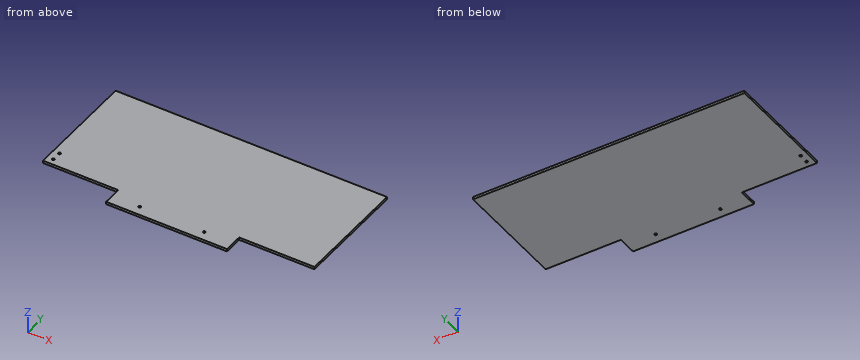
from build123d import *

# Parameters (mm, degrees)
SKETCH1_W           = 429
SKETCH1_H           = 210
BOSS_EXTRUDE1_DEPTH = 4
SKETCH2_W           = 119
SKETCH2_H           = 30
CUT_EXTRUDE1_DEPTH  = 4
SKETCH3_R           = 2
CUT_EXTRUDE2_DEPTH  = 239.854034925
SKETCH4_R           = 2
CUT_EXTRUDE3_DEPTH  = 239.854034925


with BuildPart() as part:
    # Sketch1 → Boss-Extrude1 (new body)
    with BuildSketch(Plane.XY):
        Rectangle(SKETCH1_W, SKETCH1_H)
    extrude(amount=BOSS_EXTRUDE1_DEPTH)

    # Sketch2 → Cut-Extrude1 (cut)
    with BuildSketch(Plane(origin=(0, 0, 0), x_dir=(-1, 0, 0), z_dir=(0, 0, -1))):
        with Locations((-155, -90)):
            Rectangle(SKETCH2_W, SKETCH2_H)
        with Locations((155, -90)):
            Rectangle(SKETCH2_W, SKETCH2_H)
    extrude(amount=-CUT_EXTRUDE1_DEPTH, mode=Mode.SUBTRACT)

    # Sketch3 → Cut-Extrude2 (cut, through all)
    with BuildSketch(Plane(origin=(0, 0, 0), x_dir=(-1, 0, 0), z_dir=(0, 0, -1))):
        with Locations((-49.983602513, -90)):
            Circle(SKETCH3_R)
        with Locations((52.125756906, -90)):
            Circle(SKETCH3_R)
    extrude(amount=-CUT_EXTRUDE2_DEPTH, mode=Mode.SUBTRACT)

    # Sketch4 → Cut-Extrude3 (cut, through all)
    with BuildSketch(Plane(origin=(0, 0, 0), x_dir=(-1, 0, 0), z_dir=(0, 0, -1))):
        with Locations((204.5, -65)):
            Circle(SKETCH4_R)
        with Locations((204.5, -50)):
            Circle(SKETCH4_R)
    extrude(amount=-CUT_EXTRUDE3_DEPTH, mode=Mode.SUBTRACT)


solid = part.part
Read the model definition and answer for the solid it produces. Units are mm, in the model's axes. Round coordinates to 2 decimals unless told otherwise and drop trailing zeros. Write each loop counter-clockwise with the first axis right and the second up, starting at its lowest first coordinate (ties: lowest second). Pieces come first, ordered by that corner, then holes. Notation, with made-up numbers: (87, 26.25) - (133, 26.25) arc R13 ccw to (133, 47.25) - close; hole circle Ø5 at (51.5, 52.5). An arc over 180 degrees is marked (long way). Use a Markdown table: item, result.
(1) The part is cut by section C-C (x = 151.5). Write down the section's boundary in (y, z), then the cut area to 3 significant figures.
Reported:
| item | result |
|---|---|
| outline | (-75, 0) - (105, 0) - (105, 4) - (-75, 4) - close |
| area | 720 mm2 |
(2) Each of these flat-tipped pins is pushed along its axis until it touches: pin 1 Ø2 at (y, z) = (-95, 2.5) entering from -X; pin 2 Ø2 at (x, z) = (176, 1) entering from -Y. Where does it stop, or does it pass through?
Reported:
| item | result |
|---|---|
| pin 1 | x = -95.5 |
| pin 2 | y = -75 |
(3) Straight lines are drawn through the part: line 1 along Y through (x, z) = (-204.5, 3); line 2 along X through (y, z) = (-89.5, 3.1); line 3 along Y through (x, z) = (124, 0.4). For each, find the intervals that lie inside material, in ascending order. Write a range as [from, to].
Reported:
| item | result |
|---|---|
| line 1 | [-75, -67], [-63, -52], [-48, 105] |
| line 2 | [-95.5, -54.06], [-50.19, 48.05], [51.92, 95.5] |
| line 3 | [-75, 105] |
(4) The part is cut by section A-A (z = 1). Write down the section's boundary in (x, y), then the cut area to 3 significant figures.
Reported:
| item | result |
|---|---|
| outline | (-214.5, -75) - (-95.5, -75) - (-95.5, -105) - (95.5, -105) - (95.5, -75) - (214.5, -75) - (214.5, 105) - (-214.5, 105) - close; hole circle Ø4 at (-204.5, -65); hole circle Ø4 at (-204.5, -50); hole circle Ø4 at (-52.13, -90); hole circle Ø4 at (49.98, -90) |
| area | 82,900 mm2 |
(5) The part is cut by section B-B (y = -80.5). Write down the section's boundary in (x, z).
Reported:
| item | result |
|---|---|
| outline | (-95.5, 0) - (95.5, 0) - (95.5, 4) - (-95.5, 4) - close |
